from build123d import *

# Parameters (mm, degrees)
F0_R      = 12
F1_DEPTH  = 3
F2_R      = 5.75
F3_DEPTH  = 1.2
F4_R      = 4.5
F5_DEPTH  = 8
F6_R      = 0.6
F10_DEPTH = 7
F11_W     = 1.2
F11_H     = 2.8315826069
F11_H_2   = 1.2
F11_W_2   = 2.9928033758
F12_DEPTH = 4
F13_R     = 0.4
F14_R     = 1
F15_R     = 0.2


# Not quite as in the source:
# - a feature of the source that left no trace in its solid (it failed there, or was rolled back) is left out


with BuildPart() as f1:
    # F0 (on Top) → F1 (new body)
    with BuildSketch(Plane.XY):
        Circle(F0_R)
    extrude(amount=F1_DEPTH)

    # F2 (on face) → F3 (join)
    with BuildSketch(Plane.XY.offset(3)):
        Circle(F2_R)
    extrude(amount=F3_DEPTH)

    # F4 (on face) → F5 (join)
    with BuildSketch(Plane.XY.offset(4.2)):
        Circle(F4_R)
    extrude(amount=F5_DEPTH)

    # F6 (on face) → F10 (cut)
    with BuildSketch(Plane.XY.offset(12.2)):
        Circle(F6_R)
    extrude(amount=-F10_DEPTH, mode=Mode.SUBTRACT)

    # F11 (on face) → F12 (cut)
    with BuildSketch(Plane.XY.offset(12.2)):
        with Locations((0, 2.0157913034)):
            Rectangle(F11_W, F11_H)
        Rectangle(F11_W, F11_H_2)
        with Locations((-2.0964016879, 0)):
            Rectangle(F11_W_2, F11_H_2)
        with Locations((2.0964016879, 0)):
            Rectangle(F11_W_2, F11_H_2)
        with Locations((0, -2.0157913034)):
            Rectangle(F11_W, F11_H)
    extrude(amount=-F12_DEPTH, mode=Mode.SUBTRACT)

    # F13
    f13_edges = [f1.edges().sort_by_distance(p)[0] for p in [
        (-4.5, 0, 12.2),
    ]]
    fillet(f13_edges, radius=F13_R)

    # F14
    f14_edges = [f1.edges().sort_by_distance(p)[0] for p in [
        (-12, 0, 3),
        (-12, 0, 0),
    ]]
    fillet(f14_edges, radius=F14_R)

    # F15
    f15_edges = [f1.edges().sort_by_distance(p)[0] for p in [
        (-4.1, 0, 12.2),
        (0, 3.431583, 12.2),
        (-0.6, 2.015791, 12.2),
        (-2.096402, 0.6, 12.2),
        (-3.592803, 0, 12.2),
        (-2.096402, -0.6, 12.2),
        (-0.6, -2.015791, 12.2),
        (0, -3.431583, 12.2),
        (0.6, -2.015791, 12.2),
        (2.096402, -0.6, 12.2),
        (3.592803, 0, 12.2),
        (2.096402, 0.6, 12.2),
        (0.6, 2.015791, 12.2),
        (-0.6, 0, 8.2),
    ]]
    fillet(f15_edges, radius=F15_R)


solid = f1.part
CAD build for the part. Positions are in the model's coordinates, mm. A direction names the side the tool comes from. Give positions to 0.01 mm unless a question says otherwise; leave off trailing zeros. Write each loop counter-clockwise with the first axis right and the second up, starting at its lowest first coordinate (ties: lowest second). Pieces come first, ordered by that corner, then holes. Notation, with made-up numbers: M 88,-38 L 95,-38 A16 ccw 95,-20 Z; hole C 9.5,60 d8. An arc over 180 degrees is marked long. Put each result on its own line as item: value. Start each with the question number.
(1) Mould opens along X. For faces 1 (the face through (-0.6, 2, 10)), 2 (the face through (3, -4, 4.2)), 3 (the face through (-11.99, 0.53, 1.49)), 4 (the face through (-2, -0.6, 10)) say: +X half, -X half, draft (parallel to the pull), parting line (faces both ways), or undercut.
(2) Which spindle directions (+Z, -Z, +X, -X, +Y, -Y) get a long thin tool onto all of the face, cutting with end or side? Do faces 5 (the face through (-0.6, -2, 10)), 6 (the face through (1, -1, 12.2)). Say none if no direction does.
(3) Band-saw the part on D-D, the plane z = 7. Write the cut outline in (x, y).
(4) Flat gauge pins, fed straight in: pin 1 Ø0.8 at (y, z) = (-2, 10.5) entering from -X; pin 2 Ø1 at (x, z) = (0, 10) entering from +Y; pin 3 Ø3.5 at (x, z) = (-2, 9.5) entering from -Y. Where does each tip first touch, or does it go through?
(5) Probe L1, parallel to Y at x = 0, z = 6.1; L2, parallel to Z at x = -10.5, y = -1; L3, parallel to X at y = 2.5, z = 10. List the from-to ranges inside material, lowest first.
(6) Band-saw the part on A-A, the plane z = 10.75. Write the cut outline in (x, y), and give its area (3 significant figures).
Response values:
1. face 1: undercut
1. face 2: draft
1. face 3: parting line
1. face 4: undercut
2. face 5: +Z
2. face 6: +Z, +X, -X, +Y, -Y
3. outline: C 0,0 d9; hole C 0,0 d1.2
4. pin 1: stops at x = -4.21
4. pin 2: stops at y = 4.5
4. pin 3: stops at y = -4.49
5. L1: y = -4.5 to -0.6, 0.6 to 4.5
5. L2: z = 0 to 3
5. L3: x = -3.74 to -0.6, 0.6 to 3.74
6. outline: C 0,0 d9; hole M -3.59,-0.6 L -0.6,-0.6 L -0.6,-3.43 L 0.6,-3.43 L 0.6,-0.6 L 3.59,-0.6 L 3.59,0.6 L 0.6,0.6 L 0.6,3.43 L -0.6,3.43 L -0.6,0.6 L -3.59,0.6 Z
6. area: 48.2 mm2
